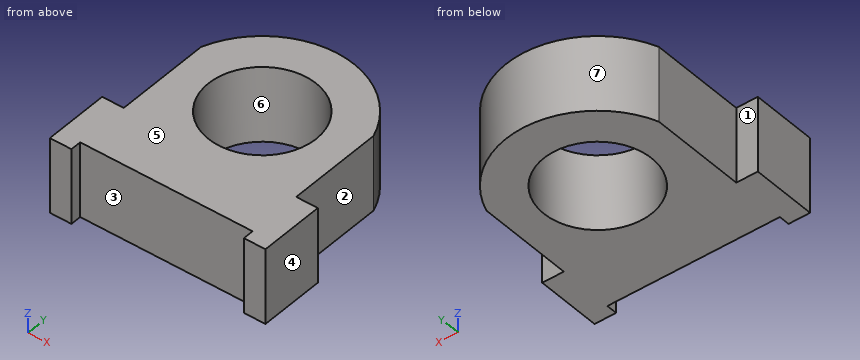
Autodesk Inventor part; units mm, degrees
ref_plane "YZ Plane" through (0, 0, 0) normal (1, 0, 0) x (0, 1, 0)
ref_plane "XZ Plane" through (0, 0, 0) normal (0, 1, 0) x (-1, 0, 0)
ref_plane "XY Plane" through (0, 0, 0) normal (0, 0, 1) x (1, 0, 0)
sketch "Sketch1" plane through (0, 0, 0) normal (0, 0, 1) x (1, 0, 0)
  line L0 (0, 0) -> (0, 152.8038)
  line L1 (-50.8, 94.6409) -> (-50.8, 38.3019)
  line L2 (-50.8, 38.3019) -> (-63.5, 38.3019)
  line L3 (-63.5, 38.3019) -> (-63.5, 0.2019)
  line L4 (-63.5, 0.2019) -> (-50.8, 0.2019)
  line L5 (-50.8, 0.2019) -> (-50.8, 6.5519)
  line L6 (-50.8, 6.5519) -> (0, 6.5519)
  line L7 (50.8, 94.6409) -> (50.8, 38.3019)
  line L8 (50.8, 38.3019) -> (63.5, 38.3019)
  line L9 (63.5, 38.3019) -> (63.5, 0.2019)
  line L10 (63.5, 0.2019) -> (50.8, 0.2019)
  line L11 (50.8, 0.2019) -> (50.8, 6.5519)
  line L12 (50.8, 6.5519) -> (0, 6.5519)
  circle A0 centre (0, 76.4019) radius 31.75
  arc A1 (50.8, 94.6409) -> (-50.8, 94.6409) centre (0, 76.4019) ccw
  dimension "d9" = 63.5
  dimension "d10" = 76.2
  dimension "d11" = 101.6
  dimension "d12" = 12.7
  dimension "d13" = 6.35
  dimension "d14" = 38.1
  dimension "d15" = 53.975
extrude "Extrusion1" add sketch "Sketch1" along normal blind 44.45 contours L6 L5 L4 L3 L2 L1 A1 L0 A0 | L0 A0 A1 L7 L8 L9 L10 L11 L12
properties part number "GuideSlider" material "Iron, Cast"
CAD build for the part. Positions are in the model's coordinates, mm. Face numbers are marked on the shaded views. A direction names the side the tool comes from. Coordinates: 2 decimals unless noted, no trailing zeros. Write each loop counter-clockwise with the first axis right and the second up, starting at its lowest first coordinate (ties: lowest second). Pieces come first, ordered by that corner, then holes. Notation, with made-up numbers: (-26, 70.25) - (31, 70.25) arc R14 cw to (31, 92.25) - close; hole circle Ø2 at (14.25, -7). An arc over 180 degrees is marked (long way). Use a Markdown table: item, result. Add a question column.
Item 1: Band-saw the part on D-D, the plane x = 45.5. Give the cut face in (y, z).
Item 2: Band-saw the part on A-A, the plane x = 0. Give the cut face in (y, z).
Item 3: Drill centre lines: L1, parallel to Y at x = 0, z = 17; L2, parallel to X at y = 93.5, z = 14; L3, parallel to X at y = 78.5, z = 39.5. Where is each one in solid material? Low to high. Write a range as from..to.
Item 4: 3-axis set-ups, long thin cutter, end or side, ignore diameter. For the marked faces 1, 2 and 3: which of +Z, -Z, +X, -X, +Y, -Y reach the whole face in a straight line?
Item 5: Flat gauge pins, fed straight in: pin 1 (5 mm diameter, centred on x = 20, z = 31, fed in from -Y); pin 2 (1 mm diameter, centred on x = 27, z = 28, fed in from +Y); pin 3 (3 mm diameter, centred on x = 39, z = 27.5, fed in from +Y). Where does each tip first touch, or does it go through?
Item 6: Band-saw the part on B-B, the plane y = 82. Give the cut face in (x, z), and give its area (3 significant figures).
Item 7: Band-saw the part on C-C, the plane z = 17. Give the cut face in (x, y) (3 decimals).
Item 8: Mould opens along X. For the marked faces 4, 5, 6 and 7 say: pulls with the +X half, pulls with the -X half, needs draft (parallel to the pull), parting line crosses it, or undercut.
Numbers:
| question | item | result |
|---|---|---|
| 1 | outline | (6.55, 0) - (105.44, 0) - (105.44, 44.45) - (6.55, 44.45) - close |
| 2 | outline | (6.55, 0) - (44.65, 0) - (44.65, 44.45) - (6.55, 44.45) - close; (108.15, 0) - (130.38, 0) - (130.38, 44.45) - (108.15, 44.45) - close |
| 3 | L1 | 6.55..44.65, 108.15..130.38 |
| 3 | L2 | -50.8..-26.75, 26.75..50.8 |
| 3 | L3 | -50.8..-31.68, 31.68..50.8 |
| 4 | face 1 | +Z, -Z, -X, +Y |
| 4 | face 2 | +Z, -Z, +X, +Y |
| 4 | face 3 | +Z, -Z, -Y |
| 5 | pin 1 | y = 6.55 |
| 5 | pin 2 | y = 123.42 |
| 5 | pin 3 | y = 115.22 |
| 6 | outline | (-50.8, 0) - (-31.25, 0) - (-31.25, 44.45) - (-50.8, 44.45) - close; (31.25, 0) - (50.8, 0) - (50.8, 44.45) - (31.25, 44.45) - close |
| 6 | area | 1,740 mm2 |
| 7 | outline | (-63.5, 0.202) - (-50.8, 0.202) - (-50.8, 6.552) - (50.8, 6.552) - (50.8, 0.202) - (63.5, 0.202) - (63.5, 38.302) - (50.8, 38.302) - (50.8, 94.641) arc R53.975 ccw to (-50.8, 94.641) - (-50.8, 38.302) - (-63.5, 38.302) - close; hole circle Ø63.5 at (0, 76.402) |
| 8 | face 4 | pulls with the +X half |
| 8 | face 5 | needs draft |
| 8 | face 6 | undercut |
| 8 | face 7 | parting line crosses it |
